```python
from build123d import *

# Parameters (mm, degrees)
EXTRUDE_THIN1_DEPTH = 500
SKETCH2_W           = 155.95
SKETCH2_H           = 20
CUT_EXTRUDE1_DEPTH  = 596.0316925
LPATTERN1_COUNT     = 14
LPATTERN1_PITCH     = 60
SKETCH3_R           = 30
CUT_EXTRUDE2_DEPTH  = 596.0316925


with BuildPart() as part:
    # Sketch1 → Extrude-Thin1 (new body, symmetric)
    with BuildSketch(Plane.XY):
        with BuildLine():
            Line((0, 0), (-205.95, 0))
            ThreePointArc((-205.95, 0), (-259.885879639, -15.792394123), (-296.786225905, -58.181582248))
            Line((-296.786225905, -58.181582248), (-539.333048865, -585.0316925))
            Line((-539.333048865, -585.0316925), (-548.416671455, -580.849850725))
            Line((-548.416671455, -580.849850725), (-305.869848496, -53.999740473))
            ThreePointArc((-305.869848496, -53.999740473), (-265.279467603, -7.371633535), (-205.95, 10))
            Line((-205.95, 10), (0, 10))
            Line((0, 10), (0, 0))
        make_face()
    extrude(amount=EXTRUDE_THIN1_DEPTH, both=True)

    # Sketch2 → Cut-Extrude1 (cut, through all)
    with BuildSketch(Plane(origin=(0, 10, 0), x_dir=(1, 0, 0), z_dir=(0, 1, 0))):
        with Locations((-97.975, 470)):
            Rectangle(SKETCH2_W, SKETCH2_H)
    cut_extrude1 = extrude(amount=-CUT_EXTRUDE1_DEPTH, mode=Mode.SUBTRACT)

    # LPattern1: Cut-Extrude1 ×14
    with Locations(*[(0, 0, i * LPATTERN1_PITCH) for i in range(1, LPATTERN1_COUNT)]):
        add(cut_extrude1, mode=Mode.SUBTRACT)

    # Sketch3 → Cut-Extrude2 (cut, through all)
    with BuildSketch(Plane(origin=(0, 10, 0), x_dir=(1, 0, 0), z_dir=(0, 1, 0))):
        with Locations((-65, -435)):
            Circle(SKETCH3_R)
    extrude(amount=-CUT_EXTRUDE2_DEPTH, mode=Mode.SUBTRACT)


solid = part.part
```
Source: CAD feature listing. Evaluate the final solid. Frame: model axes, mm. A direction names the side the tool comes from. Round coordinates to 2 decimals unless told otherwise and drop trailing zeros. Loops run counter-clockwise (first coordinate to the right, second up) from the corner with the lowest first, then second, coordinate; pieces in that order, holes last.
1. Section query A-A on z = 435. Output: boundary loops of the cut face in (x, y), and give its area (3 significant figures).
2. Access query for faces 1 (the flat face through (-193, 0, 7)), 2 (the flat face through (-334, -132, -500)). Directions: +Z, -Z, +X, -X, +Y, -Y. A direction counts if a zero-diameter tool reaches every point of the face in a straight line with its end or side. Return the directions, or none.
3. Section query C-C on z = -197. Output: boundary loops of the cut face in (x, y).
4. Mould query, pull axis X, two halves, no side actions, for faces 3 (the flat face through (-334, -132, 500)), 4 (the flat face through (-428.84, -321.11, 7)), 5 (the cylindrical face through (-259.213, -15.365, 7)), 6 (the cylindrical face through (-71.503, 5.07, 464.287)). Classes: released by +X, released by -X, zero draft, split by the parting line, or undercut.
5. Contact query for flat-ended pins moving along their axis: pin 1 (11 mm diameter, centred on y = 4, z = -414, fed in from -X); pin 2 (3 mm diameter, centred on y = -203.5, z = -103.5, fed in from +X); pin 3 (2 mm diameter, centred on x = -435, z = 3.5, fed in from -Y). Output: stop coordinate, or through.
6. Ray query, L1, parallel to X at y = -497, z = 293; L2, parallel to Y at x = -87.5, z = -456; L3, parallel to X at y = -39, z = 358. Return the intervals inside material, ascending.
7. Section query B-B on x = -65. Give the number of separate pieces and of enclosed holes in the cut face, and give its area (3 significant figures).
Answers below:
1. outline: (-548.42, -580.85) - (-539.33, -585.03) - (-296.79, -58.18) arc R100 cw to (-205.95, 0) - (-95, 0) - (-95, 10) - (-205.95, 10) arc R110 ccw to (-305.87, -54) - close; (-35, 0) - (0, 0) - (0, 10) - (-35, 10) - close
1. area: 8,460 mm2
2. face 1: +Z, -Z, +X, -Y
2. face 2: -Z, +X, -X, +Y, -Y
3. outline: (-548.42, -580.85) - (-539.33, -585.03) - (-296.79, -58.18) arc R100 cw to (-205.95, 0) - (0, 0) - (0, 10) - (-205.95, 10) arc R110 ccw to (-305.87, -54) - close
4. face 3: zero draft
4. face 4: released by -X
4. face 5: released by +X
4. face 6: undercut
5. pin 1: stops at x = -254.92
5. pin 2: stops at x = -363
5. pin 3: stops at y = -360.58
6. L1: x = -509.81 to -498.81
6. L2: y = 0 to 10
6. L3: x = -297.49 to -285.19
7. separate pieces: 16
7. enclosed holes: 0
7. area: 6,600 mm2
